```python
from build123d import *

# Parameters (mm, degrees)
F0_W     = 2
F0_H     = 18
F1_DEPTH = 18
F2_R     = 1
F3_DEPTH = 25
F4_R     = 3
F5_R     = 1
F6_R     = 1
F7_R     = 8.99999


# Not quite as in the source:
# - a fillet or chamfer is up to 0.001 mm smaller than in the source, because OpenCascade refuses the exact size


with BuildPart() as f1:
    # F0 (on Top) → F1 (new body)
    with BuildSketch(Plane.XY):
        Polygon((-1, 5), (-1, -25), (1, -25), (1, 25), (-1, 25), align=None)
        Polygon((1, -25), (-1, -25), (-1, -27), (19, -27), (19, -25), (17, -25), align=None)
        Polygon((-15, 25), (-1, 5), (-1, 25), align=None)
        Polygon((-1, 25), (1, 25), (1, 27), (-15, 27), (-15, 25), align=None)
        with Locations((18, -16)):
            Rectangle(F0_W, F0_H)
    extrude(amount=F1_DEPTH)

    # F2 (on face) → F3 (cut)
    with BuildSketch(Plane(origin=(0, 27, 0), x_dir=(-1, 0, 0), z_dir=(0, 1, 0))):
        with Locations((9, 9)):
            Circle(F2_R)
        with Locations((13, 9)):
            Circle(F2_R)
    extrude(amount=-F3_DEPTH, mode=Mode.SUBTRACT)

    # F4
    f4_edges = [f1.edges().sort_by_distance(p)[0] for p in [
        (19, -27, 9),
    ]]
    fillet(f4_edges, radius=F4_R)

    # F5
    f5_edges = [f1.edges().sort_by_distance(p)[0] for p in [
        (17, -25, 9),
    ]]
    fillet(f5_edges, radius=F5_R)

    # F6
    f6_edges = [f1.edges().sort_by_distance(p)[0] for p in [
        (-1, -27, 9),
    ]]
    fillet(f6_edges, radius=F6_R)

    # F7 (radius 9 in the source; OpenCascade refuses exactly that, so slightly less here)
    f7_edges = [f1.edges().sort_by_distance(p)[0] for p in [
        (18, -7, 18),
        (18, -7, 0),
    ]]
    fillet(f7_edges, radius=F7_R)


solid = f1.part
```
Verification items for the finished model (mm, model axes). A direction names the side the tool comes from. Give positions to 0.01 mm unless a question says otherwise; leave off trailing zeros. Write each loop counter-clockwise with the first axis right and the second up, starting at its lowest first coordinate (ties: lowest second). Pieces come first, ordered by that corner, then holes. Notation, with made-up numbers: (21, 39.25) - (39, 39.25) arc R29 cw to (39, 59.25) - close; hole circle Ø5 at (37, -32). An arc over 180 degrees is marked (long way). Put each result on its own line as item: value.
Q1. Scan lines: probe 1 along X at (y, z) = (25, 9); probe 2 along Z at (x, y) = (-13, 25); probe 3 along X at (y, z) = (21.5, 9). Record each from-to range of solid material in increasing order. Write a range as from..to.
Result:
probe 1: -15..-14, -12..-10, -8..1
probe 2: 0..8, 10..18
probe 3: -12..-10, -8..1
Q2. Section check C-C on y = -6. Record the cut outline in (x, z).
Result:
outline: (-1, 0) - (1, 0) - (1, 18) - (-1, 18) - close
Q3. Mould release check, pull along Z, two halves, no side actions. Record for faces 1 (the face through (17, -16, 9)), 2 (the face through (-12, 25, 9)), 3 (the face through (-8, 22, 9)), 4 (the face through (-1, 6, 0)): released by +Z, released by -Z, zero draft, split by the parting line, or undercut.
Result:
face 1: zero draft
face 2: undercut
face 3: undercut
face 4: released by -Z
Q4. Section check B-B on z = 12. Record the cut outline in (x, y).
Result:
outline: (-15, 25) - (-1, 5) - (-1, -26) arc R1 ccw to (0, -27) - (16, -27) arc R3 ccw to (19, -24) - (19, -7.51) - (17, -7.51) - (17, -24) arc R1 cw to (16, -25) - (1, -25) - (1, 27) - (-15, 27) - close
Q5. Section check A-A on x = -13. Record the cut outline in (y, z), and give its area (3 significant figures).
Result:
outline: (22.14, 0) - (27, 0) - (27, 8) - (22.14, 8) - close; (22.14, 10) - (27, 10) - (27, 18) - (22.14, 18) - close
area: 77.7 mm2
Q6. Section check D-D on x = 6. Record the cut outline in (y, z), and give its area (3 significant figures).
Result:
outline: (-27, 0) - (-25, 0) - (-25, 18) - (-27, 18) - close
area: 36.0 mm2
Q7. Set-up check for faces 5 (the face through (18.014, -9.566, 15.294)), 6 (the face through (18.014, -9.706, 2.566)), 7 (the face through (18.1, -26.14, 9.13)), 8 (the face through (9, -25, 9)), 9 (the face through (-1, -10, 9)): record each of +Z, -Z, +X, -X, +Y, -Y from which the full face is reachable in a straight line by a thin tool's end or side.
Result:
face 5: +Z, +X, +Y
face 6: -Z, +X, +Y
face 7: +Z, -Z, +X, -Y
face 8: +Z, -Z, +Y
face 9: +Z, -Z, -X, -Y
Q8. Depth check by flat-ended pin: P1, Ø5, axis at x = -0.5, y = -2, coming from the -Z side; P2, Ø5, axis at x = 7, z = 13.5, coming from the +Y side; P3, Ø8.5, axis at y = -12.5, z = 9, coming from the -X side; P4, Ø5, axis at y = -0.5, z = 2, coming from the +X side. Enter the tip coordinate at first touch or a pass-through.
Result:
P1: z = 0
P2: y = -25
P3: x = -1
P4: x = 1
